Geometry check sheet. Reference: the model listing, model coordinates, mm. Face numbers are marked on the shaded views. A direction names the side the tool comes from. Give positions to 0.01 mm unless a question says otherwise; leave off trailing zeros. Order: outer loops, then holes, each group sorted by start corner. A loop starts at its lowest first (then second) coordinate and runs counter-clockwise, first axis right, second up.
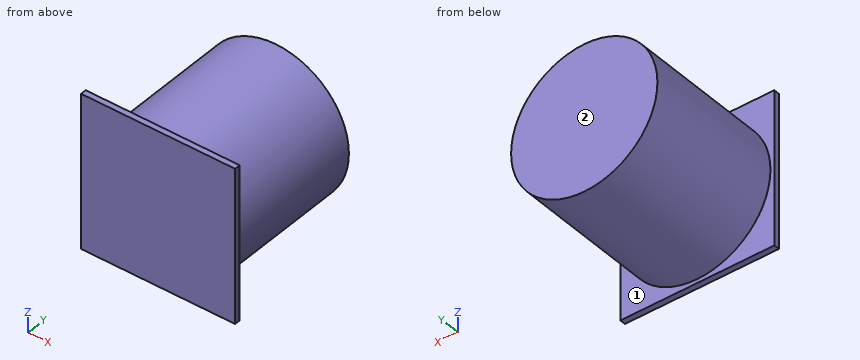
```python
from build123d import *

# Parameters (mm, degrees)
SKETCH1_W           = 80
SKETCH1_H           = 80
BOSS_EXTRUDE1_DEPTH = 3
SKETCH3_R           = 38
SKETCH3_R_2         = 35
EXTRUDE_THIN1_DEPTH = 74


with BuildPart() as part:
    # Sketch1 → Boss-Extrude1 (new body)
    with BuildSketch(Plane(origin=(0, 0, 0), x_dir=(1, 0, 0), z_dir=(0, 1, 0))):
        with Locations((40, 0)):
            Rectangle(SKETCH1_W, SKETCH1_H)
    extrude(amount=BOSS_EXTRUDE1_DEPTH)

    # Sketch3 → Extrude-Thin1 (add)
    with BuildSketch(Plane(origin=(0, 3, 0), x_dir=(1, 0, 0), z_dir=(0, 1, 0))):
        with Locations((40, 0)):
            Circle(SKETCH3_R)
        with Locations((40, 0)):
            Circle(SKETCH3_R_2, mode=Mode.SUBTRACT)
    extrude(amount=EXTRUDE_THIN1_DEPTH)

    # Sketch7 → Revolve5 (revolve)
    with BuildSketch(Plane.XY):
        Polygon((40, 77), (2, 77), (2, 36), (40, 74), align=None)
    revolve(axis=Axis((40, 77, 0), (0, -1, 0)))


solid = part.part
```
Q1. Cross-section at B-B, the plane y = 24. Record the boundary of the cut face in (x, z), and give its area (3 significant figures).
Q2. Thickness scan on L1, parallel to Z at x = 40, y = 22; L2, parallel to X at y = 16.5, z = 0; L3, parallel to X at y = 43, z = 13.5. Record the ranges inside material, lowest first.
Q3. Access from +Z, -Z, +X, -X, +Y, -Y to the whole of each face (thin tool, end or side, straight path). Record for the marked faces 1 and 2.
Q4. Cross-section at A-A, the plane y = 56.5. Record the boundary of the cut face in (x, z).
Q5. Gauge pin test, flat ends, axial feed: P1, Ø2, axis at x = 38.5, z = -2, coming from the -Y side; P2, Ø12, axis at x = 59.5, y = 67, coming from the -Z side; P3, Ø1, axis at x = 37.5, y = 64, coming from the +Z side; P4, Ø6, axis at y = 37, z = 9, coming from the +X side. Record the tip position at first contact, or that the pin passes through.
Answers follow:
1. outline: circle Ø76 at (40, 0); hole circle Ø70 at (40, 0)
1. area: 688 mm2
2. L1: z = -38 to -35, 35 to 38
2. L2: x = 2 to 5, 75 to 78
2. L3: x = 4.48 to 12.09, 67.91 to 75.52
3. face 1: +Y
3. face 2: +Z, -Z, +X, -X, +Y
4. outline: circle Ø76 at (40, 0); hole circle Ø35 at (40, 0)
5. P1: stops at y = 0
5. P2: stops at z = -35.52
5. P3: stops at z = 37.95
5. P4: stops at x = 77.52
